from build123d import *

# Parameters (mm, degrees)
SKETCH1_R           = 42.055
SKETCH1_R_2         = 9.525
SKETCH1_R_3         = 4
BOSS_EXTRUDE1_DEPTH = 5
SKETCH2_R           = 15
BOSS_EXTRUDE2_DEPTH = 30
SKETCH3_R           = 9.525
CUT_EXTRUDE1_DEPTH  = 72.674584408


with BuildPart() as part:
    # Sketch1 → Boss-Extrude1 (new, symmetric)
    with BuildSketch(Plane.XY):
        Circle(SKETCH1_R)
        Circle(SKETCH1_R_2, mode=Mode.SUBTRACT)
        with Locations((0, 30)):
            Circle(SKETCH1_R_3, mode=Mode.SUBTRACT)
        with Locations((-30, 0)):
            Circle(SKETCH1_R_3, mode=Mode.SUBTRACT)
        with Locations(Location((0, -30, 0), (0, 0, 180))):
            Circle(SKETCH1_R_3, mode=Mode.SUBTRACT)
        with Locations(Location((30, 0, 0), (0, 0, 180))):
            Circle(SKETCH1_R_3, mode=Mode.SUBTRACT)
    extrude(amount=BOSS_EXTRUDE1_DEPTH, both=True)

    # Sketch2 → Boss-Extrude2 (add)
    with BuildSketch(Plane.XY.offset(5)):
        Circle(SKETCH2_R)
    extrude(amount=BOSS_EXTRUDE2_DEPTH)

    # Sketch3 → Cut-Extrude1 (cut, through all)
    with BuildSketch(Plane.XY.offset(35)):
        Circle(SKETCH3_R)
    extrude(amount=-CUT_EXTRUDE1_DEPTH, mode=Mode.SUBTRACT)


solid = part.part
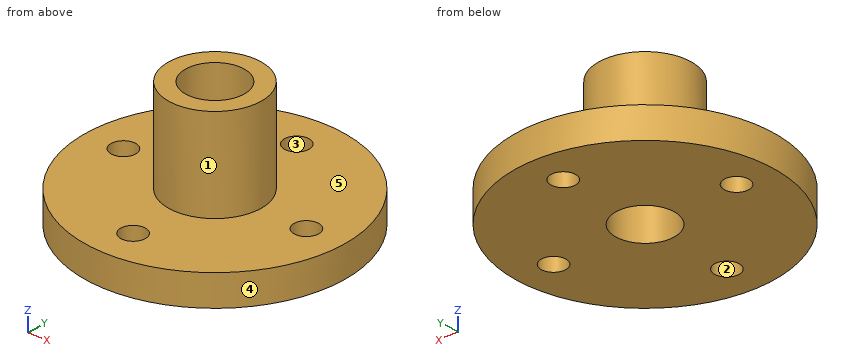
Geometry check sheet. Reference: the model listing, model coordinates, mm. Face numbers are marked on the shaded views. A direction names the side the tool comes from. Give positions to 0.01 mm unless a question says otherwise; leave off trailing zeros. Loops run counter-clockwise (first coordinate to the right, second up) from the corner with the lowest first, then second, coordinate; pieces in that order, holes last.
(1) Section check A-A on y = 0. Record the cut outline in (x, z) (3 decimals), then the cut area to 3 significant figures.
From the geometry:
outline: (-42.055, -5) - (-34, -5) - (-34, 5) - (-42.055, 5) - close; (-26, -5) - (-9.525, -5) - (-9.525, 35) - (-15, 35) - (-15, 5) - (-26, 5) - close; (9.525, -5) - (26, -5) - (26, 5) - (15, 5) - (15, 35) - (9.525, 35) - close; (34, -5) - (42.055, -5) - (42.055, 5) - (34, 5) - close
area: 819 mm2
(2) Release check for a two-part mould opening along X. For the marked faces 3, 4 and 5 record: released by +X, released by -X, zero draft, split by the parting line, or undercut.
From the geometry:
face 3: undercut
face 4: split by the parting line
face 5: zero draft
(3) Thickness scan on L1, parallel to Y at x = 0, z = 2.5 (3 decimals); L2, parallel to Z at x = -9, y = 14; L3, parallel to X at y = 7, z = 23. Record the ranges inside material, lowest first.
From the geometry:
L1: y = -42.055 to -34, -26 to -9.525, 9.525 to 26, 34 to 42.055
L2: z = -5 to 5
L3: x = -13.27 to -6.46, 6.46 to 13.27
(4) Section check C-C on z = 1.5. Record the cut outline in (x, y) (3 decimals), then the cut area to 3 significant figures.
From the geometry:
outline: circle Ø84.11 at (0, 0); hole circle Ø8 at (-30, 0); hole circle Ø19.05 at (0, 0); hole circle Ø8 at (0, -30); hole circle Ø8 at (0, 30); hole circle Ø8 at (30, 0)
area: 5,070 mm2
(5) Depth check by flat-ended pin: pin 1 Ø25 at (x, y) = (0, 0) entering from -Z; pin 2 Ø2 at (y, z) = (-12.5, -0.5) entering from -X; pin 3 Ø5 at (y, z) = (-6.5, 10.5) entering from -X; pin 4 Ø4 at (y, z) = (27.5, 1) entering from -X. Enter the tip coordinate at first touch or a pass-through.
From the geometry:
pin 1: stops at z = -5
pin 2: stops at x = -40.45
pin 3: stops at x = -14.46
pin 4: stops at x = -33.44
(6) Set-up check for the marked faces 1 and 2: record each of +Z, -Z, +X, -X, +Y, -Y from which the full face is reachable in a straight line by a thin tool's end or side.
From the geometry:
face 1: +Z
face 2: +Z, -Z
(7) Section check D-D on x = -31. Record the cut outline in (y, z).
From the geometry:
outline: (-28.42, -5) - (-3.87, -5) - (-3.87, 5) - (-28.42, 5) - close; (3.87, -5) - (28.42, -5) - (28.42, 5) - (3.87, 5) - close
